Here's how the part is built. I have some questions about the finished solid (model axes, mm). Give positions to 0.01 mm unless a question says otherwise; leave off trailing zeros. Put each result on its own line as item: value. Start each with the question number.
from build123d import *

# Parameters (mm, degrees)
SKIZZE1_W                       = 300
SKIZZE1_H                       = 140
AUFSATZ_LINEAR_AUSTRAGEN2_DEPTH = 6
SKIZZE2_R                       = 2.5
SCHNITT_LINEAR_AUSTRAGEN1_DEPTH = 6
LINEARES_MUSTER1_COUNT          = 15
LINEARES_MUSTER1_PITCH          = 20
LINEARES_MUSTER1_COUNT_DIR2     = 7
LINEARES_MUSTER1_PITCH_DIR2     = 20
SKIZZE5_R                       = 1.5
SCHNITT_LINEAR_AUSTRAGEN3_DEPTH = 10
SKIZZE4_R                       = 1.51
CORTAR_EXTRUIR1_DEPTH           = 10
MATRIZL1_COUNT                  = 2
MATRIZL1_PITCH                  = 100
MATRIZL1_COUNT_DIR2             = 2
MATRIZL1_PITCH_DIR2             = 20
MATRIZL2_COUNT                  = 2
MATRIZL2_PITCH                  = 100
MATRIZL2_COUNT_DIR2             = 2
MATRIZL2_PITCH_DIR2             = 280
CROQUIS1_R                      = 1.5
CORTAR_EXTRUIR2_DEPTH           = 10
MATRIZL3_COUNT                  = 2
MATRIZL3_PITCH                  = 100
MATRIZL3_COUNT_DIR2             = 2
MATRIZL3_PITCH_DIR2             = 20
CROQUIS2_R                      = 1.5
CORTAR_EXTRUIR3_DEPTH           = 10
MATRIZL4_COUNT                  = 4
MATRIZL4_PITCH                  = 20
MATRIZL4_COUNT_DIR2             = 2
MATRIZL4_PITCH_DIR2             = 100


with BuildPart() as part:
    # Skizze1 → Aufsatz-Linear austragen2 (new body)
    with BuildSketch(Plane.XY):
        Rectangle(SKIZZE1_W, SKIZZE1_H)
    extrude(amount=AUFSATZ_LINEAR_AUSTRAGEN2_DEPTH)

    # Skizze2 → Schnitt-Linear austragen1 (cut)
    with BuildSketch(Plane(origin=(0, 0, 0), x_dir=(-1, 0, 0), z_dir=(0, 0, -1))):
        with Locations((-140, 60)):
            Circle(SKIZZE2_R)
    schnitt_linear_austragen1 = extrude(amount=-SCHNITT_LINEAR_AUSTRAGEN1_DEPTH, mode=Mode.SUBTRACT)

    # Lineares Muster1: Schnitt-Linear austragen1 15 × 7
    with Locations(*[(-i * LINEARES_MUSTER1_PITCH, -j * LINEARES_MUSTER1_PITCH_DIR2, 0) for i in range(LINEARES_MUSTER1_COUNT) for j in range(LINEARES_MUSTER1_COUNT_DIR2) if (i, j) != (0, 0)]):
        add(schnitt_linear_austragen1, mode=Mode.SUBTRACT)

    # Skizze5 → Schnitt-Linear austragen3 (cut)
    with BuildSketch(Plane(origin=(0, 0, 0), x_dir=(-1, 0, 0), z_dir=(0, 0, -1))):
        with Locations((-140, 50)):
            Circle(SKIZZE5_R)
    schnitt_linear_austragen3 = extrude(amount=-SCHNITT_LINEAR_AUSTRAGEN3_DEPTH, mode=Mode.SUBTRACT)

    # Skizze4 → Cortar-Extruir1 (cut)
    with BuildSketch(Plane(origin=(0, 0, 0), x_dir=(-1, 0, 0), z_dir=(0, 0, -1))):
        with Locations((-110, 50.3739212)):
            Circle(SKIZZE4_R)
    cortar_extruir1 = extrude(amount=-CORTAR_EXTRUIR1_DEPTH, mode=Mode.SUBTRACT)

    # MatrizL1: Cortar-Extruir1 2 × 2
    with Locations(*[(-j * MATRIZL1_PITCH_DIR2, -i * MATRIZL1_PITCH, 0) for i in range(MATRIZL1_COUNT) for j in range(MATRIZL1_COUNT_DIR2) if (i, j) != (0, 0)]):
        add(cortar_extruir1, mode=Mode.SUBTRACT)

    # MatrizL2: Schnitt-Linear austragen3 2 × 2
    with Locations(*[(-j * MATRIZL2_PITCH_DIR2, -i * MATRIZL2_PITCH, 0) for i in range(MATRIZL2_COUNT) for j in range(MATRIZL2_COUNT_DIR2) if (i, j) != (0, 0)]):
        add(schnitt_linear_austragen3, mode=Mode.SUBTRACT)

    # Croquis1 → Cortar-Extruir2 (cut)
    with BuildSketch(Plane(origin=(0, 0, 0), x_dir=(-1, 0, 0), z_dir=(0, 0, -1))):
        with Locations((110, 50)):
            Circle(CROQUIS1_R)
    cortar_extruir2 = extrude(amount=-CORTAR_EXTRUIR2_DEPTH, mode=Mode.SUBTRACT)

    # MatrizL3: Cortar-Extruir2 2 × 2
    with Locations(*[(j * MATRIZL3_PITCH_DIR2, -i * MATRIZL3_PITCH, 0) for i in range(MATRIZL3_COUNT) for j in range(MATRIZL3_COUNT_DIR2) if (i, j) != (0, 0)]):
        add(cortar_extruir2, mode=Mode.SUBTRACT)

    # Croquis2 → Cortar-Extruir3 (cut)
    with BuildSketch(Plane(origin=(0, 0, 0), x_dir=(-1, 0, 0), z_dir=(0, 0, -1))):
        with Locations((30, 50)):
            Circle(CROQUIS2_R)
    cortar_extruir3 = extrude(amount=-CORTAR_EXTRUIR3_DEPTH, mode=Mode.SUBTRACT)

    # MatrizL4: Cortar-Extruir3 4 × 2
    with Locations(*[(i * MATRIZL4_PITCH, -j * MATRIZL4_PITCH_DIR2, 0) for i in range(MATRIZL4_COUNT) for j in range(MATRIZL4_COUNT_DIR2) if (i, j) != (0, 0)]):
        add(cortar_extruir3, mode=Mode.SUBTRACT)


solid = part.part
1) I want a section at A-A, the plane z = 1.65. State how many separate pieces and enclosed holes the cut face has, and give its area (3 significant figures).
2) I'm going to push a flat-ended pin straight in: pin 1 Ø2.5 at (x, y) = (-10, -50) entering from -Z. Where does the tip first touch, or does it pass through?
3) Thinking about a two-plate mould opening in Y: for faces 1 (the flat face through (150, -1, 3)), 2 (the cylindrical face through (82.5, -39.9, 3)), which applies, released by +Y, released by -Y, zero draft, split by the parting line, or undercut?
Established:
1. separate pieces: 1
1. enclosed holes: 125
1. area: 39,800 mm2
2. pin 1: passes through
3. face 1: zero draft
3. face 2: undercut
